Job drawing, mm, ordinate dimensions from the low corner. One solid piece. A direction names the side the tool comes from. Round coordinates to 2 decimals unless told otherwise and drop trailing zeros. Write each loop counter-clockwise with the first axis right and the second up, starting at its lowest first coordinate (ties: lowest second). Pieces come first, ordered by that corner, then holes. Notation, with made-up numbers: M 20.25,87 L 52.25,87 A29 ccw 52.25,115 Z; hole C 5.5,57.5 d8. An arc over 180 degrees is marked long. Answer as a JSON object with one key per item and string values. Group by question number.
1. Band-saw the part on D-D, the plane x = 16.5. Write the cut outline in (y, z).
2. Which spindle directions (+Z, -Z, +X, -X, +Y, -Y) get a long thin tool onto all of the face, cutting with end or side? Do the marked faces 1, 2 and 3. Say none if no direction does.
3. Drop flat-ended pins along their axis: pin 1 (6 mm diameter, centred on x = 14, z = 2.5, fed in from +Y); pin 2 (1.2 mm diameter, centred on y = 26, z = 10.5, fed in from -X); pin 3 (4 mm diameter, centred on x = 11, y = 6, fed in from -Z). Give the stop position or say it passes through.
4. Band-saw the part on B-B, the plane y = 6. Write the cut outline in (x, z).
5. Two-plate mould, pull along X, no slides. Class the marked faces 4, 5 and 6: +X half, -X half, draft (parallel to the pull), parting line (faces both ways), or undercut.
6. Drill centre lines: line 1 (X direction, y = 32.4, z = 9); line 2 (X direction, y = 30.65, z = 9); line 3 (Z direction, x = 2, y = 23.35). Where is each one in solid material? Low to high. Write a range as from..to.
7. Band-saw the part on A-A, the plane x = 30.5. Write the cut outline in (y, z) (1 decimal).
8. Band-saw the part on C-C, the plane x = 2. Write the cut outline in (y, z), plus the area to 3 significant figures.
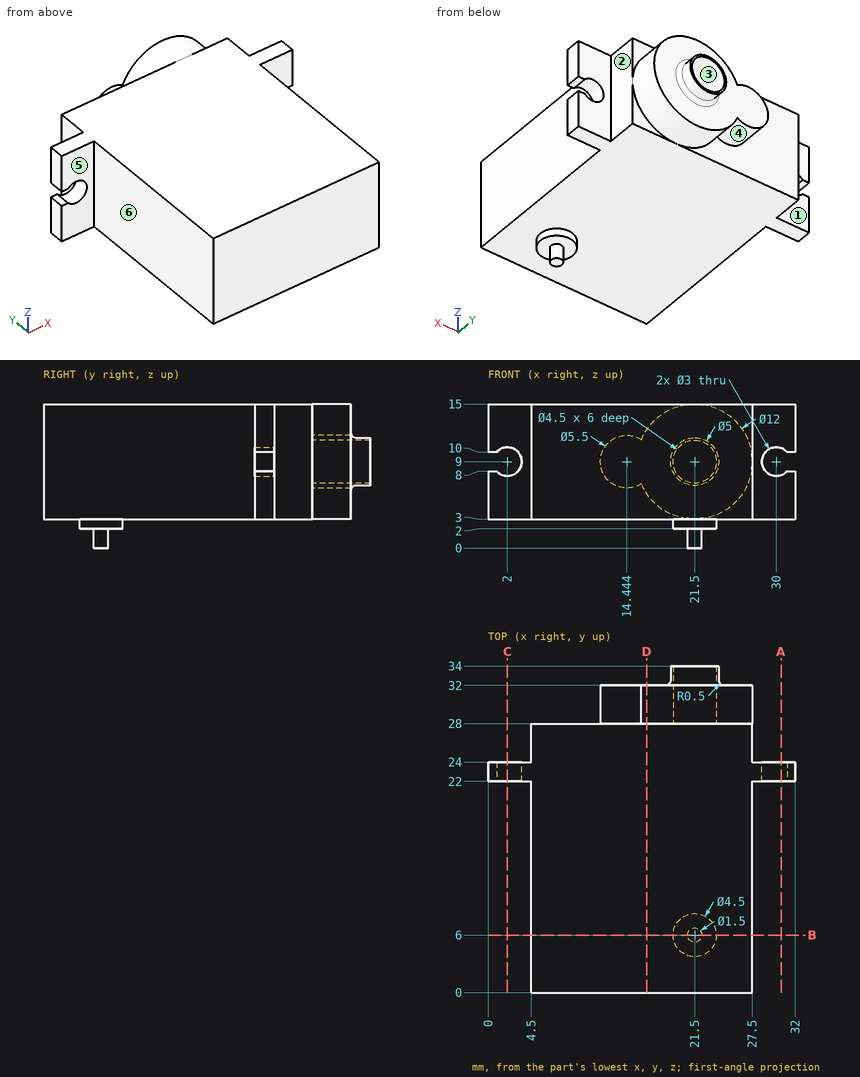
Worked answers:
{
 "1": {"outline": "M 0,3 L 28,3 L 28,5.68 L 32,5.68 L 32,12.32 L 28,12.32 L 28,15 L 0,15 Z"},
 "2": {"face 1": "+Z, -Z, -X, +Y", "face 2": "+Z, -Z, +X, +Y", "face 3": "+Y"},
 "3": {"pin 1": "stops at y = 28", "pin 2": "stops at x = 4.5", "pin 3": "stops at z = 3"},
 "4": {"outline": "M 4.5,3 L 19.25,3 L 19.25,2 L 20.75,2 L 20.75,0 L 22.25,0 L 22.25,2 L 23.75,2 L 23.75,3 L 27.5,3 L 27.5,15 L 4.5,15 Z"},
 "5": {"face 4": "undercut", "face 5": "draft", "face 6": "-X half"},
 "6": {"line 1": "x = 18.99..19.25, 23.75..24.01", "line 2": "x = 11.69..19.25, 23.75..27.5", "line 3": "z = 3..7.5, 10.5..15"},
 "7": {"outline": "M 22,3 L 24,3 L 24,7.6 L 22,7.6 Z; M 22,10.4 L 24,10.4 L 24,15 L 22,15 Z"},
 "8": {"outline": "M 22,3 L 24,3 L 24,7.5 L 22,7.5 Z; M 22,10.5 L 24,10.5 L 24,15 L 22,15 Z", "area": "18.0 mm^2"}
}
